Source: CAD feature listing. Evaluate the final solid. Frame: model axes, mm. Give positions to 0.01 mm unless a question says otherwise; leave off trailing zeros. Loops run counter-clockwise (first coordinate to the right, second up) from the corner with the lowest first, then second, coordinate; pieces in that order, holes last. Notation, with made-up numbers: M 28.25,22.25 L 46.25,22.25 A19 cw 46.25,43.25 Z; hole C 52.5,16.5 d6. An arc over 180 degrees is marked long. Answer in a Markdown table with one row per item.
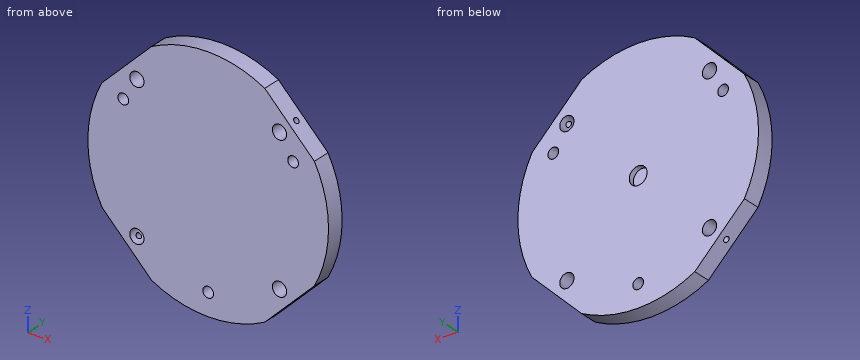
```python
from build123d import *

# Parameters (mm, degrees)
SKETCH1_R                  = 67.5
BOSS_EXTRUDE1_DEPTH        = 10
F_6_0MM_DOWEL_HOLE1_D      = 6
CUT_EXTRUDE1_DEPTH         = 96.981769102
CUT_EXTRUDE1_DEPTH_BACK    = 96.981769102
SKETCH4_R                  = 4
CUT_EXTRUDE_THIN1_DEPTH    = 96.981769102
F_3_0MM_DOWEL_HOLE1_REACH  = 162.34
F_3_0MM_DOWEL_HOLE1_BORE_R = 1.5
CIRPATTERN1_COUNT          = 4
CUT_EXTRUDE2_DEPTH         = 96.981769113
CUT_EXTRUDE2_DEPTH_BACK    = 3
SKETCH8_R                  = 5


with BuildPart() as part:
    # Sketch1 → Boss-Extrude1 (new body)
    with BuildSketch(Plane(origin=(0, 0, 0), x_dir=(1, 0, 0), z_dir=(0, 1, 0))):
        with Locations(Location((0, 0, 0), (0, 0, 270))):
            Circle(SKETCH1_R)
    extrude(amount=BOSS_EXTRUDE1_DEPTH)

    # Ø6.0mm Dowel Hole1 (through all)
    with Locations(Plane(origin=(0, 10, 0), x_dir=(1, 0, 0), z_dir=(0, 1, 0))):
        with Locations((0, 55), (47.631397208, -27.5), (-47.631397208, -27.5)):
            Hole(F_6_0MM_DOWEL_HOLE1_D / 2)

    # Sketch4 → Cut-Extrude1 (cut, two sides: drawn at the far end of the back side and taken through both)
    with BuildSketch(Plane(origin=(0, 10, 0), x_dir=(1, 0, 0), z_dir=(0, 1, 0)).offset(-CUT_EXTRUDE1_DEPTH_BACK)):
        with Locations(Location((-40, 40, 0), (0, 0, 270))):
            Circle(SKETCH4_R)
        with Locations(Location((40, 40, 0), (0, 0, 270))):
            Circle(SKETCH4_R)
        with Locations(Location((40, -40, 0), (0, 0, 270))):
            Circle(SKETCH4_R)
        with Locations(Location((-40, -40, 0), (0, 0, 270))):
            Circle(SKETCH4_R)
    extrude(amount=CUT_EXTRUDE1_DEPTH + CUT_EXTRUDE1_DEPTH_BACK, mode=Mode.SUBTRACT)

    # Sketch5 → Cut-Extrude-Thin1 (cut, through all)
    with BuildSketch(Plane(origin=(0, 10, 0), x_dir=(1, 0, 0), z_dir=(0, 1, 0))):
        Polygon((-31.743671291, 59.570037208), (-59.570037208, 31.743671291), (-66.64110502, 38.814739103), (-38.814739103, 66.64110502), align=None)
        Polygon((59.570037208, 31.743671291), (31.743671291, 59.570037208), (38.814739103, 66.64110502), (66.64110502, 38.814739103), align=None)
        Polygon((31.743671291, -59.570037208), (59.570037208, -31.743671291), (66.64110502, -38.814739103), (38.814739103, -66.64110502), align=None)
        Polygon((-59.570037208, -31.743671291), (-31.743671291, -59.570037208), (-38.814739103, -66.64110502), (-66.64110502, -38.814739103), align=None)
    extrude(amount=-CUT_EXTRUDE_THIN1_DEPTH, mode=Mode.SUBTRACT)

    # Ø3.0mm Dowel Hole1 bore → Ø3.0mm Dowel Hole1 (cut, up to next)
    with BuildSketch(Plane(origin=(45.656854249, 0, 45.656854249), x_dir=(0.7071067811865479, 0, -0.7071067811865471), z_dir=(0.7071067811865471, 0, 0.7071067811865479)), mode=Mode.PRIVATE) as f_3_0mm_dowel_hole1_sk1:
        with Locations((0, 5)):
            Circle(F_3_0MM_DOWEL_HOLE1_BORE_R)
    f_3_0mm_dowel_hole1_tool1 = extrude(f_3_0mm_dowel_hole1_sk1.sketch, amount=-F_3_0MM_DOWEL_HOLE1_REACH, mode=Mode.PRIVATE) & part.part
    f_3_0mm_dowel_hole1 = f_3_0mm_dowel_hole1_tool1.solids().sort_by_distance((45.656854, 5, 45.656854))[0]
    add(f_3_0mm_dowel_hole1, mode=Mode.SUBTRACT)

    # CirPattern1: Ø3.0mm Dowel Hole1 ×4 about axis
    cirpattern1_axis = Axis((0, 10, 0), (0, -1, 0))
    for i in range(1, CIRPATTERN1_COUNT):
        add(f_3_0mm_dowel_hole1.rotate(cirpattern1_axis, i * 360 / CIRPATTERN1_COUNT), mode=Mode.SUBTRACT)

    # Sketch8 → Cut-Extrude2 (cut, two sides: drawn at the far end of the back side and taken through both)
    with BuildSketch(Plane(origin=(0, 10, 0), x_dir=(1, 0, 0), z_dir=(0, 1, 0)).offset(-CUT_EXTRUDE2_DEPTH_BACK)):
        with Locations(Location((0, 0, 0), (0, 0, 90))):
            Circle(SKETCH8_R)
    extrude(amount=CUT_EXTRUDE2_DEPTH + CUT_EXTRUDE2_DEPTH_BACK, mode=Mode.SUBTRACT)


solid = part.part
```
Q1. Section query D-D (z = 27.5). Output: boundary loops of the cut face in (x, y).
Values follow:
| item | result |
|---|---|
| outline | M -61.64,0 L -50.63,0 L -50.63,10 L -61.64,10 Z; M -44.63,0 L 44.63,0 L 44.63,10 L -44.63,10 Z; M 50.63,0 L 61.64,0 L 61.64,10 L 50.63,10 Z |
Q2. Section query B-B (z = 0). Output: boundary loops of the cut face in (x, y).
Values follow:
| item | result |
|---|---|
| outline | M -67.5,0 L 67.5,0 L 67.5,10 L 5,10 L 5,7 L -5,7 L -5,10 L -67.5,10 Z |
Q3. Section query A-A (x = 0). Output: boundary loops of the cut face in (y, z), plus the area to 3 significant figures.
Values follow:
| item | result |
|---|---|
| outline | M 0,-67.5 L 10,-67.5 L 10,-58 L 0,-58 Z; M 0,-52 L 10,-52 L 10,-5 L 7,-5 L 7,5 L 10,5 L 10,67.5 L 0,67.5 Z |
| area | 1,260 mm^2 |
Q4. Contact query for flat-ended pins moving along their axis: pin 1 Ø2 at (y, z) = (8.5, 0) entering from +X; pin 2 Ø4 at (x, y) = (-24, 2.5) entering from -Z; pin 3 Ø6.5 at (x, z) = (-40, -40) entering from +Y; pin 4 Ø1 at (x, y) = (-15.5, 7) entering from -Z. Output: stop coordinate, or through.
Values follow:
| item | result |
|---|---|
| pin 1 | x = 67.5 |
| pin 2 | z = -63.81 |
| pin 3 | through |
| pin 4 | z = -65.81 |
Q5. Section query C-C (x = 40). Output: boundary loops of the cut face in (y, z).
Values follow:
| item | result |
|---|---|
| outline | M 0,-51.31 L 10,-51.31 L 10,-44 L 0,-44 Z; M 0,-36 L 10,-36 L 10,36 L 0,36 Z; M 0,44 L 10,44 L 10,51.31 L 0,51.31 Z |
Q6. Ray query, probe 1 along X at (y, z) = (4.5, -40); probe 2 along X at (y, z) = (3.75, 41.5); probe 3 along X at (y, z) = (6.5, -55). Return the intervals inside material, ascending. Write a range as from..to.
Values follow:
| item | result |
|---|---|
| probe 1 | -51.31..-44, -36..36, 44..51.31 |
| probe 2 | -49.81..-43.71, -36.29..36.29, 43.71..49.81 |
| probe 3 | -36.31..-3, 3..36.31 |
